```python
from build123d import *

# Parameters (mm, degrees)
F0_W     = 76.2
F0_H     = 177.8
F0_R     = 5.588
F0_R_2   = 15.875
F1_DEPTH = 4.826
F2_SIZE  = 12.7
F3_W     = 63.5
F3_H     = 6.35
F4_DEPTH = 6.35


with BuildPart() as f1:
    # F0 (on Top) → F1 (new body)
    with BuildSketch(Plane.XY):
        with Locations((0, -63.5)):
            Rectangle(F0_W, F0_H)
        with Locations((-25.4, -127)):
            Circle(F0_R, mode=Mode.SUBTRACT)
        with Locations((25.4, -127)):
            Circle(F0_R, mode=Mode.SUBTRACT)
        Circle(F0_R_2, mode=Mode.SUBTRACT)
    extrude(amount=F1_DEPTH)

    # F2
    f2_edges = [f1.edges().sort_by_distance(p)[0] for p in [
        (38.1, 25.4, 2.413),
        (-38.1, 25.4, 2.413),
    ]]
    chamfer(f2_edges, length=F2_SIZE)

    # F3 (on face) → F4 (join)
    with BuildSketch(Plane(origin=(0, 0, 0), x_dir=(1, 0, 0), z_dir=(0, 0, -1))):
        with Locations((0, 96.901)):
            Rectangle(F3_W, F3_H)
    extrude(amount=F4_DEPTH)


solid = f1.part
```
Input: part model. Units: mm. Frame: model coordinates. A direction names the side the tool comes from. Coordinates: 2 decimals unless noted, no trailing zeros. Loops run counter-clockwise (first coordinate to the right, second up) from the corner with the lowest first, then second, coordinate; pieces in that order, holes last. Notation, with made-up numbers: M 54.25,66.5 L 89.25,66.5 A21 ccw 89.25,80.5 Z; hole C 81,0.25 d10. An arc over 180 degrees is marked long. Answer in a Markdown table with one row per item.
1. Reachability of faces 4 (the flat face through (-31.75, -97, -3)), 5 (the flat face through (0, -93.726, -3)), 6 (the flat face through (0, -100.076, -3)), 7 (the flat face through (31.75, -97, -3)), 8 (the flat face through (-1, -152.4, 2)) from +Z, -Z, +X, -X, +Y, -Y: full face, straight path, thin tool, end or side. Return the list, or none.
Response:
| item | result |
|---|---|
| face 4 | -Z, -X, +Y, -Y |
| face 5 | -Z, +X, -X, +Y |
| face 6 | -Z, +X, -X, -Y |
| face 7 | -Z, +X, +Y, -Y |
| face 8 | +Z, -Z, +X, -X, -Y |
2. Section D-D, the plane y = -127. Output: boundary loops of the cut face in (x, z), then the cut area to 3 significant figures.
Response:
| item | result |
|---|---|
| outline | M -38.1,0 L -30.99,0 L -30.99,4.83 L -38.1,4.83 Z; M -19.81,0 L 19.81,0 L 19.81,4.83 L -19.81,4.83 Z; M 30.99,0 L 38.1,0 L 38.1,4.83 L 30.99,4.83 Z |
| area | 260 mm2 |
3. Draft query along X for faces 1 (the flat face through (-1, -62, 0)), 2 (the cylindrical face through (-26.611, -132.455, 2.379)), 3 (the flat face through (31.8, 19, 2.4)). Return one class per face: pulls with the +X half, pulls with the -X half, needs draft (parallel to the pull), parting line crosses it, or undercut.
Response:
| item | result |
|---|---|
| face 1 | needs draft |
| face 2 | undercut |
| face 3 | pulls with the +X half |
4. First-contact query: pin 1 (1.5 mm diameter, centred on x = 6, z = -1.5, fed in from -Y); pin 2 (5 mm diameter, centred on x = -8.5, z = -4.5, fed in from +Y); pin 3 (3 mm diameter, centred on y = -98, z = -4, fed in from +X). Flat tips, straight axial feed; report the tip coordinate or a pass-through.
Response:
| item | result |
|---|---|
| pin 1 | stops at y = -100.08 |
| pin 2 | stops at y = -93.73 |
| pin 3 | stops at x = 31.75 |
5. Material intervals for line 1 (Y direction, x = 0, z = 2) (3 decimals); line 2 (Z direction, x = -10, y = 17.5); line 3 (Y direction, x = -25.4, z = 3.35), sorted ascending.
Response:
| item | result |
|---|---|
| line 1 | y = -152.4 to -15.875, 15.875 to 25.4 |
| line 2 | z = 0 to 4.83 |
| line 3 | y = -152.4 to -132.59, -121.41 to 25.4 |
6. Section A-A, the plane y = 0. Output: boundary loops of the cut face in (x, z) (3 decimals), then the cut area to 3 significant figures.
Response:
| item | result |
|---|---|
| outline | M -38.1,0 L -15.875,0 L -15.875,4.826 L -38.1,4.826 Z; M 15.875,0 L 38.1,0 L 38.1,4.826 L 15.875,4.826 Z |
| area | 215 mm2 |
7. Section B-B, the plane x = -2.5. Output: boundary loops of the cut face in (y, z).
Response:
| item | result |
|---|---|
| outline | M -152.4,0 L -100.08,0 L -100.08,-6.35 L -93.73,-6.35 L -93.73,0 L -15.68,0 L -15.68,4.83 L -152.4,4.83 Z; M 15.68,0 L 25.4,0 L 25.4,4.83 L 15.68,4.83 Z |
8. Section C-C, the plane z = 2.5. Output: boundary loops of the cut face in (x, y) (3 decimals).
Response:
| item | result |
|---|---|
| outline | M -38.1,-152.4 L 38.1,-152.4 L 38.1,12.7 L 25.4,25.4 L -25.4,25.4 L -38.1,12.7 Z; hole C -25.4,-127 d11.176; hole C 0,0 d31.75; hole C 25.4,-127 d11.176 |
